Geometry check sheet. Reference: the model listing, model coordinates, mm. Coordinates: 2 decimals unless noted, no trailing zeros. Loops run counter-clockwise (first coordinate to the right, second up) from the corner with the lowest first, then second, coordinate; pieces in that order, holes last. Notation, with made-up numbers: (85.25, 56) - (106.25, 56) arc R25 cw to (106.25, 86) - close; hole circle Ø8 at (70.25, 54). An arc over 180 degrees is marked (long way). One line per item, written item: value.
from build123d import *

# Parameters (mm, degrees)
BOSS_EXTRUDE1_DEPTH     = 101.6
SKETCH2_R               = 3.175
CUT_EXTRUDE1_DEPTH      = 930.148
CUT_EXTRUDE2_DEPTH      = 129.032
CUT_EXTRUDE2_DEPTH_BACK = 167.132
SKETCH3_R               = 3.175


with BuildPart() as part:
    # Sketch1 → Boss-Extrude1 (new body)
    with BuildSketch(Plane.XY):
        Polygon((0, 949.461691672), (0, 1270), (203.850246616, 0), (152.4, 0), align=None)
    extrude(amount=BOSS_EXTRUDE1_DEPTH)

    # Sketch2 → Cut-Extrude1 (cut)
    with BuildSketch(Plane.ZY):
        with Locations(Location((50.8, 1213.824708718, 0), (0, 0, 270))):
            Circle(SKETCH2_R)
        with Locations(Location((50.8, 1092.198474258, 0), (0, 0, 270))):
            Circle(SKETCH2_R)
    extrude(amount=-CUT_EXTRUDE1_DEPTH, mode=Mode.SUBTRACT)

    # Sketch3 → Cut-Extrude2 (cut, two sides: drawn at the far end of the back side and taken through both)
    with BuildSketch(Plane(origin=(101.925123308, 101.925123308, 0), x_dir=(0, 0, -1), z_dir=(-0.7071067811865487, -0.7071067811865465, 0)).offset(-CUT_EXTRUDE2_DEPTH_BACK)):
        with Locations(Location((-67.733333333, 125.953482591, 0), (0, 0, 270))):
            Circle(SKETCH3_R)
        with Locations(Location((-33.866666667, 125.953482591, 0), (0, 0, 270))):
            Circle(SKETCH3_R)
    extrude(amount=CUT_EXTRUDE2_DEPTH + CUT_EXTRUDE2_DEPTH_BACK, mode=Mode.SUBTRACT)


solid = part.part
(1) Cross-section at B-B on y = 388. Record the cut outline in (x, z), and give its area (3 significant figures).
Reply:
outline: (90.12, 0) - (141.57, 0) - (141.57, 101.6) - (90.12, 101.6) - close
area: 5,230 mm2
(2) Material ranges on probe 1 along X at (y, z) = (853.5, 78); probe 2 along X at (y, z) = (961, 70.5), recorded low to high. Write a range as from..to.
Reply:
probe 1: 15.4..66.85
probe 2: 0..49.6
(3) Cross-section at A-A on z = 12. Record the cut outline in (x, y).
Reply:
outline: (0, 949.46) - (152.4, 0) - (203.85, 0) - (0, 1270) - close
(4) Go/stop test with flat-tipped pins: pin 1 Ø4 at (y, z) = (494, 86.5) entering from -X; pin 2 Ø4 at (y, z) = (243.5, 27.5) entering from -X; pin 3 Ø7.5 at (y, z) = (1213.82, 50.8) entering from +X. Record where each tip stops, or that it passes through.
Reply:
pin 1: x = 72.79
pin 2: x = 112.99
pin 3: x = 9.62
(5) Release check for a two-part mould opening along X. For faces 1 (the face through (0, 1107, 50)), 2 (the face through (95, 544, 0)), 3 (the face through (186.94, 13.1, 66.78)) record: pulls with the +X half, pulls with the -X half, needs draft (parallel to the pull), parting line crosses it, or undercut.
Reply:
face 1: pulls with the -X half
face 2: needs draft
face 3: undercut
